Can you work these out from the model? Positions are in its coordinate system, mm. Face numbers are marked on the shaded views. A direction names the side the tool comes from. Coordinates: 2 decimals unless noted, no trailing zeros. Loops run counter-clockwise (first coordinate to the right, second up) from the corner with the lowest first, then second, coordinate; pieces in that order, holes last.
```python
from build123d import *

# Parameters (mm, degrees)
SKETCH19_W          = 115
SKETCH19_H          = 10
BOSS_EXTRUDE4_DEPTH = 3
SKETCH22_R          = 2.5
BOSS_EXTRUDE5_DEPTH = 1


with BuildPart() as part:
    # Sketch19 → Boss-Extrude4 (new body, symmetric)
    with BuildSketch(Plane.XY):
        Rectangle(SKETCH19_W, SKETCH19_H)
    boss_extrude4 = extrude(amount=BOSS_EXTRUDE4_DEPTH, both=True)

    # Sketch22 → Boss-Extrude5 (add, symmetric)
    with BuildSketch(Plane.XY):
        with BuildLine():
            Line((57.5, 5), (67.5, 5))
            ThreePointArc((67.5, 5), (72.5, 0), (67.5, -5))
            Line((67.5, -5), (57.5, -5))
            Line((57.5, -5), (57.5, 5))
        make_face()
        with Locations((67.5, 0)):
            Circle(SKETCH22_R, mode=Mode.SUBTRACT)
    boss_extrude5 = extrude(amount=BOSS_EXTRUDE5_DEPTH, both=True)

    # Mirror1: Boss-Extrude4, Boss-Extrude5 across plane
    add(boss_extrude4.mirror(Plane(origin=(0, 0, 0), x_dir=(0, 0, 1), z_dir=(1, 0, 0))))
    add(boss_extrude5.mirror(Plane(origin=(0, 0, 0), x_dir=(0, 0, 1), z_dir=(1, 0, 0))))


solid = part.part
```
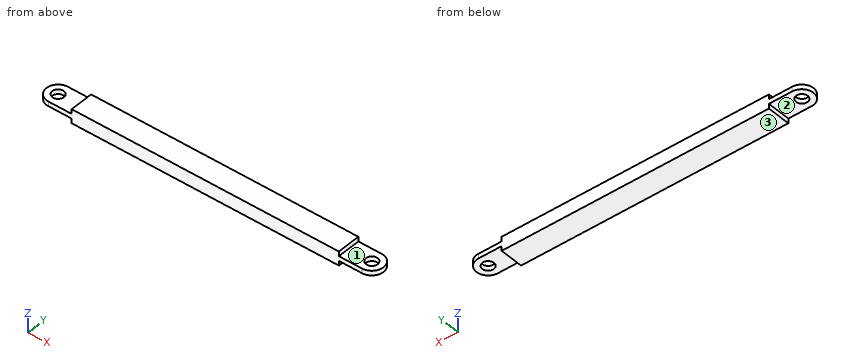
(1) Which directions (+Z, -Z, +X, -X, +Y, -Y) give clear straight access to the entire face, cutting with the end or side of a thin tool? Please do the marked faces 1, 2 and 3.
Check values:
face 1: +Z, +X, +Y, -Y
face 2: -Z, -X, +Y, -Y
face 3: -Z, +X, -X, +Y, -Y
(2) I'm going to push flat-ended pins straight in: pin 1 (5 mm diameter, centred on x = -66, y = -1.5, fed in from +Z); pin 2 (0.6 mm diameter, centred on y = 0.5, z = 2, fed in from -X); pin 3 (3 mm diameter, centred on y = -3, z = -1.5, fed in from +X); pin 4 (4.5 mm diameter, centred on x = 67.5, y = 0, fed in from -Z). Where does each tip first touch, or does it pass through?
Check values:
pin 1: stops at z = 1
pin 2: stops at x = -57.5
pin 3: stops at x = 72.24
pin 4: passes through
(3) I want a section at A-A on y = 0. Write out the boundary of the cut face in (x, z), then the cut area to 3 significant figures.
Check values:
outline: (-72.5, -1) - (-70, -1) - (-70, 1) - (-72.5, 1) - close; (-65, -1) - (-57.5, -1) - (-57.5, -3) - (57.5, -3) - (57.5, -1) - (65, -1) - (65, 1) - (57.5, 1) - (57.5, 3) - (-57.5, 3) - (-57.5, 1) - (-65, 1) - close; (70, -1) - (72.5, -1) - (72.5, 1) - (70, 1) - close
area: 730 mm2
(4) If I drill on probe 1 along Y at (x, z) = (-67.5, 0.35); probe 2 along X at (y, z) = (-0.5, 1.65); probe 3 along Z at (x, y) = (63, 0.5), over which ranges is the centre line in solid material (lowest first)?
Check values:
probe 1: y = -5 to -2.5, 2.5 to 5
probe 2: x = -57.5 to 57.5
probe 3: z = -1 to 1
